from build123d import *

# Parameters (mm, degrees)
SKETCH1_R                = 62.4
SKETCH1_R_2              = 42
BOSS_EXTRUDE1_DEPTH      = 0.725
BOSS_EXTRUDE2_DEPTH      = 0.725
CUT_EXTRUDE2_DEPTH       = 93.663561474
FILLET1_R                = 1.5
CIRPATTERN1_COUNT        = 6
FILLET1_OF_CIRPATTERN1_R = 1.5
BOSS_EXTRUDE3_START      = 0.725
SKETCH5_R                = 60.5
SKETCH5_R_2              = 42
BOSS_EXTRUDE3_DEPTH      = 0.5
BOSS_EXTRUDE5_START      = -1.225
SKETCH5_4_R              = 60.5
SKETCH5_4_R_2            = 42
BOSS_EXTRUDE5_DEPTH      = 0.5


with BuildPart() as part:
    # Sketch1 → Boss-Extrude1 (new, symmetric)
    with BuildSketch(Plane(origin=(0, 0, 0), x_dir=(1, 0, 0), z_dir=(0, 1, 0))):
        with Locations(Location((0, 0, 0), (0, 0, 270))):
            Circle(SKETCH1_R)
        with Locations(Location((0, 0, 0), (0, 0, 270))):
            Circle(SKETCH1_R_2, mode=Mode.SUBTRACT)
    boss_extrude1 = extrude(amount=BOSS_EXTRUDE1_DEPTH, both=True)

    # Sketch2 → Boss-Extrude2 (add, symmetric)
    with BuildSketch(Plane(origin=(0, 0, 0), x_dir=(1, 0, 0), z_dir=(0, 1, 0))):
        with BuildLine():
            Line((-6, 68.5), (6, 68.5))
            Line((6, 68.5), (6, 62.110868614))
            ThreePointArc((6, 62.110868614), (0, 62.4), (-6, 62.110868614))
            Line((-6, 62.110868614), (-6, 68.5))
        make_face()
    boss_extrude2 = extrude(amount=BOSS_EXTRUDE2_DEPTH, both=True)

    # Sketch4 → Cut-Extrude2 (cut, symmetric)
    with BuildSketch(Plane(origin=(0, 0, 0), x_dir=(1, 0, 0), z_dir=(0, 1, 0))):
        with BuildLine():
            ThreePointArc((-6, 62.110868614), (-9.588011618, 61.658981772), (-13.143819841, 61))
            Line((-13.143819841, 61), (-6, 61))
            Line((-6, 61), (-6, 62.110868614))
        make_face()
        with BuildLine():
            Line((6, 61), (13.143819841, 61))
            ThreePointArc((13.143819841, 61), (9.588011618, 61.658981772), (6, 62.110868614))
            Line((6, 62.110868614), (6, 61))
        make_face()
    cut_extrude2 = extrude(amount=CUT_EXTRUDE2_DEPTH, both=True, mode=Mode.SUBTRACT)

    # Fillet1
    fillet1_edges = [part.edges().sort_by_distance(p)[0] for p in [
        (-6, 0, -61),
        (6, 0, -61),
    ]]
    fillet(fillet1_edges, radius=FILLET1_R)

    # CirPattern1: Boss-Extrude1, Boss-Extrude2, Cut-Extrude2 ×6 about axis
    cirpattern1_axis = Axis((0, 0, 0), (0, 1, 0))
    add([boss_extrude1.rotate(cirpattern1_axis, i * 360 / CIRPATTERN1_COUNT) for i in range(1, CIRPATTERN1_COUNT)])
    add([boss_extrude2.rotate(cirpattern1_axis, i * 360 / CIRPATTERN1_COUNT) for i in range(1, CIRPATTERN1_COUNT)])
    add([cut_extrude2.rotate(cirpattern1_axis, i * 360 / CIRPATTERN1_COUNT) for i in range(1, CIRPATTERN1_COUNT)], mode=Mode.SUBTRACT)

    # Fillet1 of CirPattern1
    fillet1_of_cirpattern1_edges = [part.edges().sort_by_distance(p)[0] for p in [
        (-55.827549631, 0, -25.303847577),
        (-49.827549631, 0, -35.696152423),
        (-49.827549631, 0, 35.696152423),
        (-55.827549631, 0, 25.303847577),
        (6, 0, 61),
        (-6, 0, 61),
        (55.827549631, 0, 25.303847577),
        (49.827549631, 0, 35.696152423),
        (49.827549631, 0, -35.696152423),
        (55.827549631, 0, -25.303847577),
    ]]
    fillet(fillet1_of_cirpattern1_edges, radius=FILLET1_OF_CIRPATTERN1_R)

    # Sketch5 → Boss-Extrude3 (add)
    with BuildSketch(Plane(origin=(0, 0, 0), x_dir=(1, 0, 0), z_dir=(0, 1, 0)).offset(BOSS_EXTRUDE3_START)):
        with Locations(Location((0, 0, 0), (0, 0, 270))):
            Circle(SKETCH5_R)
        with Locations(Location((0, 0, 0), (0, 0, 270))):
            Circle(SKETCH5_R_2, mode=Mode.SUBTRACT)
    extrude(amount=BOSS_EXTRUDE3_DEPTH)

    # Sketch5<4> → Boss-Extrude5 (add)
    with BuildSketch(Plane(origin=(0, 0, 0), x_dir=(1, 0, 0), z_dir=(0, 1, 0)).offset(BOSS_EXTRUDE5_START)):
        with Locations(Location((0, 0, 0), (0, 0, 270))):
            Circle(SKETCH5_4_R)
        with Locations(Location((0, 0, 0), (0, 0, 270))):
            Circle(SKETCH5_4_R_2, mode=Mode.SUBTRACT)
    extrude(amount=BOSS_EXTRUDE5_DEPTH)


solid = part.part
Check sheet for the modelled part. Datum: model origin and axes. Units: mm. A direction names the side the tool comes from. Coordinates: 2 decimals unless noted, no trailing zeros. Loops run counter-clockwise (first coordinate to the right, second up) from the corner with the lowest first, then second, coordinate; pieces in that order, holes last. Notation, with made-up numbers: (0, 80) -> (12, 80) arc R23 cw to (12, 119) -> close; hole circle Ø1 at (71.5, 24.5). An arc over 180 degrees is marked (long way). Answer in a Markdown table with one row per item.
1. Release check for a two-part mould opening along Z. For faces 1 (the face through (12.62, -0.02, 40.06)), 2 (the face through (53.761, 0.01, 37.967)), 3 (the face through (53.688, -0.01, -37.925)) record: released by +Z, released by -Z, zero draft, split by the parting line, or undercut.
Check values:
| item | result |
|---|---|
| face 1 | undercut |
| face 2 | released by +Z |
| face 3 | released by -Z |
2. Go/stop test with flat-tipped pins: pin 1 (1.2 mm diameter, centred on y = -0.5, z = -66.5, fed in from -X); pin 2 (1 mm diameter, centred on x = 13, y = 0.5, fed in from +Z); pin 3 (0.7 mm diameter, centred on y = -0.5, z = -67, fed in from +X). Record where each tip stops, or that it passes through.
Check values:
| item | result |
|---|---|
| pin 1 | stops at x = -6 |
| pin 2 | stops at z = 61 |
| pin 3 | stops at x = 6 |
3. Access from +Z, -Z, +X, -X, +Y, -Y to the whole of each face (thin tool, end or side, straight path). Record for faces 4 (the face through (56, 0.725, 25)), 5 (the face through (-47.65, -0.01, 39.47)), 6 (the face through (-47.69, 0.01, -39.4)).
Check values:
| item | result |
|---|---|
| face 4 | +Y |
| face 5 | +Z, +Y, -Y |
| face 6 | -Z, +Y, -Y |
4. Sectioned sample at C-C, the plane z = 49.5. Record the boundary of the cut face in (x, y) (3 decimals), then the cut area to 3 significant figures.
Check values:
| item | result |
|---|---|
| outline | (-37.994, -0.725) -> (-34.785, -0.725) -> (-34.785, -1.225) -> (34.785, -1.225) -> (34.785, -0.725) -> (37.994, -0.725) -> (37.994, 0.725) -> (34.785, 0.725) -> (34.785, 1.225) -> (-34.785, 1.225) -> (-34.785, 0.725) -> (-37.994, 0.725) -> close |
| area | 180 mm2 |
5. Sectioned sample at B-B, the plane x = 15.5. Record the boundary of the cut face in (y, z) (3 decimals), then the cut area to 3 significant figures.
Check values:
| item | result |
|---|---|
| outline | (-1.225, -58.481) -> (-0.725, -58.481) -> (-0.725, -60.444) -> (0.725, -60.444) -> (0.725, -58.481) -> (1.225, -58.481) -> (1.225, -39.035) -> (-1.225, -39.035) -> close; (-1.225, 39.035) -> (1.225, 39.035) -> (1.225, 58.481) -> (0.725, 58.481) -> (0.725, 60.444) -> (-0.725, 60.444) -> (-0.725, 58.481) -> (-1.225, 58.481) -> close |
| area | 101 mm2 |
6. Material ranges on line 1 along X through (y, z) = (0.25, 0); line 2 along X through (y, z) = (0, -38); line 3 along X through (y, z) = (-0.2, 23), recorded low to high. Write a range as [from, to].
Check values:
| item | result |
|---|---|
| line 1 | x = [-62.4, -42], [42, 62.4] |
| line 2 | x = [-57.16, -53.82], [-48.5, -17.89], [17.89, 48.5], [53.82, 57.16] |
| line 3 | x = [-57.16, -35.14], [35.14, 57.16] |
7. Sectioned sample at D-D, the plane z = -47.5. Record the boundary of the cut face in (x, y) (3 decimals), then the cut area to 3 significant figures.
Check values:
| item | result |
|---|---|
| outline | (-40.466, -0.725) -> (-37.47, -0.725) -> (-37.47, -1.225) -> (37.47, -1.225) -> (37.47, -0.725) -> (40.466, -0.725) -> (40.466, 0.725) -> (37.47, 0.725) -> (37.47, 1.225) -> (-37.47, 1.225) -> (-37.47, 0.725) -> (-40.466, 0.725) -> close |
| area | 192 mm2 |
8. Sectioned sample at A-A, the plane z = 0. Record the boundary of the cut face in (x, y) (3 decimals), then the cut area to 3 significant figures.
Check values:
| item | result |
|---|---|
| outline | (-62.4, -0.725) -> (-60.5, -0.725) -> (-60.5, -1.225) -> (-42, -1.225) -> (-42, 1.225) -> (-60.5, 1.225) -> (-60.5, 0.725) -> (-62.4, 0.725) -> close; (42, -1.225) -> (60.5, -1.225) -> (60.5, -0.725) -> (62.4, -0.725) -> (62.4, 0.725) -> (60.5, 0.725) -> (60.5, 1.225) -> (42, 1.225) -> close |
| area | 96.2 mm2 |
